For this review, take the finished solid that the model builds, in its own axes (mm). Face numbers are marked on the shaded views. Round coordinates to 2 decimals unless told otherwise and drop trailing zeros. One line per item, written item: value. Start each with the question number.
Q1. Mouldability with a two-part tool opening along Z and no side actions: class the marked faces 1 and 2 as +Z half, -Z half, draft (parallel to the pull), parting line (faces both ways), or undercut.
Q2. For probe 1 along Y at (x, z) = (-85, 21); probe 2 along Y at (x, z) = (-85.5, 17) (3 decimals); probe 3 along X at (y, z) = (101.6, 23.5) (3 decimals), list the stretches that pass through material, from the lowest coordinate up.
Q3. Clearance check with a flat-ended pin moving along its axis: pin 1 Ø8 at (x, y) = (-57, 1651) entering from -Z. State where the tip first meets the part, or that it passes through.
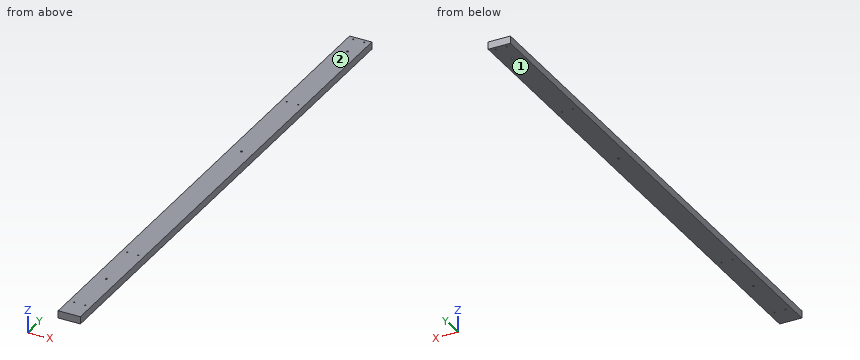
Autodesk Inventor part; units mm, degrees
ref_plane "YZ Plane" through (0, 0, 0) normal (1, 0, 0) x (0, 1, 0)
ref_plane "XZ Plane" through (0, 0, 0) normal (0, 1, 0) x (-1, 0, 0)
ref_plane "XY Plane" through (0, 0, 0) normal (0, 0, 1) x (1, 0, 0)
sketch "Sketch1" plane through (0, 0, 0) normal (0, 1, 0) x (-1, 0, 0)
  line L0 (0, 0) -> (114, 0)
  line L1 (114, 0) -> (114, 38)
  line L2 (114, 38) -> (0, 38)
  line L3 (0, 38) -> (0, 0)
  dimension "d0" = 114
  dimension "d1" = 38
extrude "Extrusion1" add sketch "Sketch1" along normal blind 2794
sketch "Sketch3" plane through (-114, 0, 38) normal (0, 0, 1) x (1, 0, 0)
  line L0 (0, 0) -> (114, 0)
  line L1 (0, 0) -> (0, 2794)
  circle A0 centre (28.5, 101.6) radius 5.7238
  circle A1 centre (85.5, 101.6) radius 5.7238
  circle A2 centre (28.5, 609.6) radius 5.7238
  circle A3 centre (85.5, 609.6) radius 5.7238
  dimension "d28" = 101.6
  dimension "d29" = 28.5
  dimension "d32" = 57
  dimension "d35" = 508
hole "rimArm" at (-85.5, 609.6, 38) at (-28.5, 609.6, 38) at (-85.5, 101.6, 38) at (-28.5, 101.6, 38) direction (0, 0, -1) diameter 6.35 end through all
sketch "Sketch4" plane through (-114, 0, 38) normal (0, 0, 1) x (1, 0, 0)
  line L0 (0, 2794) -> (114, 2794)
  line L1 (0, 0) -> (0, 2794)
  circle A0 centre (28.5, 2774.95) radius 4.8454
  circle A1 centre (85.5, 2774.95) radius 4.8454
  circle A2 centre (28.5, 2139.95) radius 4.8454
  circle A3 centre (85.5, 2139.95) radius 4.8454
  dimension "d45" = 19.05
  dimension "d48" = 57
  dimension "d51" = 635
  dimension "d71" = 28.5
hole "screenArm" at (-85.5, 2774.95, 38) at (-28.5, 2774.95, 38) at (-28.5, 2139.95, 38) at (-85.5, 2139.95, 38) direction (0, 0, -1) diameter 6.7564 end through all
sketch "Sketch5" plane through (-114, 0, 38) normal (0, 0, 1) x (1, 0, 0)
  line L0 (0, 0) -> (114, 0)
  line L1 (0, 2794) -> (114, 2794)
  circle A0 centre (57, 2667) radius 8.4367
  circle A1 centre (57, 1651) radius 12.5456
  circle A2 centre (57, 355.6) radius 11.5895
  line L2 (0, 0) -> (0, 2794)
  dimension "d61" = 127
  dimension "d62" = 355.6
  dimension "d70" = 1651
  dimension "d72" = 57
  dimension "d73" = 57
  dimension "d74" = 57
hole "poleAttach" at (-57, 2667, 38) at (-57, 1651, 38) at (-57, 355.6, 38) direction (0, 0, -1) diameter 10.0838 end through all
equation "\"d29\" = 0.25 * d0"
equation "\"d32\" = 0.5 * d0"
equation "\"d48\" = 0.5 * d0"
equation "\"d71\" = 0.25 * d0"
equation "\"d72\" = 0.5 * d0"
equation "\"d73\" = 0.5 * d0"
equation "\"d74\" = 0.5 * d0"
properties part number "2p2psv" material "Wood (Cherry)"
Result set:
1. face 1: -Z half
1. face 2: +Z half
2. probe 1: y = 0 to 98.46, 104.74 to 606.46, 612.74 to 2136.61, 2143.29 to 2771.61, 2778.29 to 2794
2. probe 2: y = 0 to 98.425, 104.775 to 606.425, 612.775 to 2136.572, 2143.328 to 2771.572, 2778.328 to 2794
2. probe 3: x = -114 to -88.675, -82.325 to -31.675, -25.325 to 0
3. pin 1: passes through
